Input: dimensioned drawing with shaded views. Units: mm. Origin: part minimum x, y, z. Coordinates: 2 decimals unless noted, no trailing zeros. Order: outer loops, then holes, each group sorted by start corner. A loop starts at its lowest first (then second) coordinate and runs counter-clockwise, first axis right, second up.
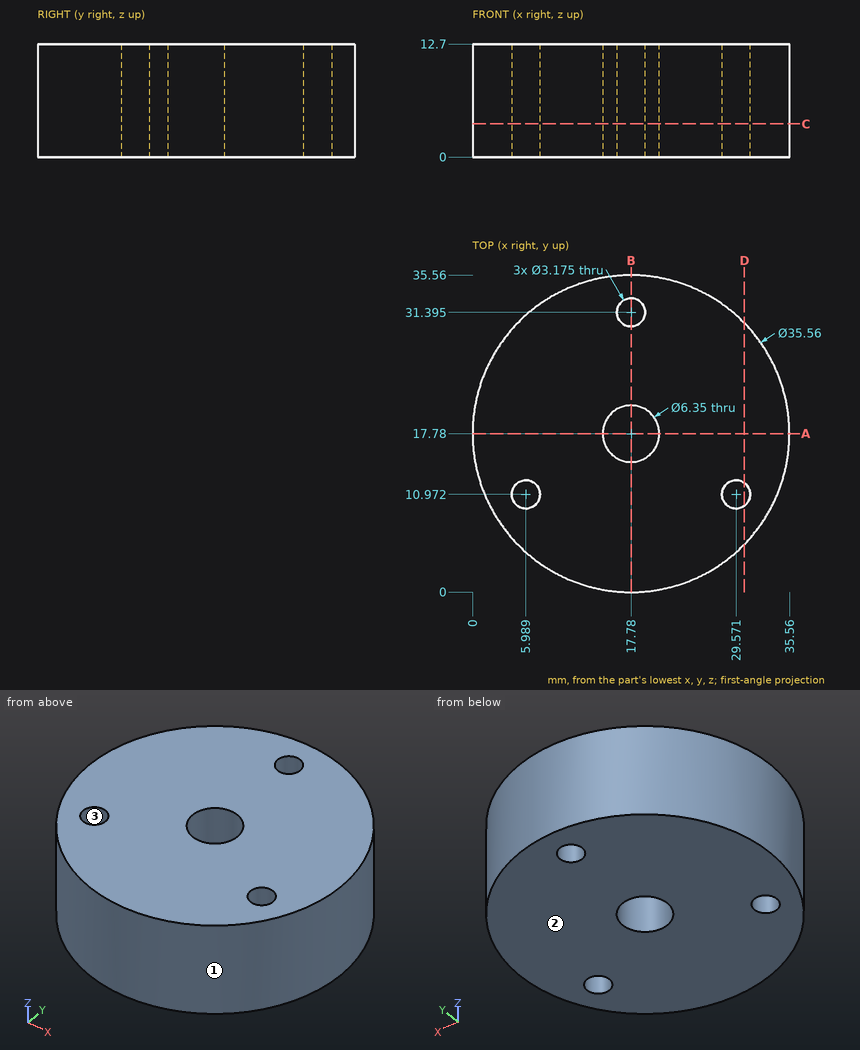
1. Section query A-A on y = 17.78. Return loops of the section in (x, z) (1 decimal), plus the area to 3 significant figures.
Findings:
outline: (0, 0) - (14.6, 0) - (14.6, 12.7) - (0, 12.7) - close; (21, 0) - (35.6, 0) - (35.6, 12.7) - (21, 12.7) - close
area: 371 mm2
2. Section query C-C on z = 3.75. Count the separate pieces of the cut face and the enclosed holes in it, plus the area to 3 significant figures.
Findings:
separate pieces: 1
enclosed holes: 4
area: 938 mm2
3. Pin query (flat end, axial travel): P1, Ø4, axis at x = 4.5, z = 3.5, coming from the +Y side; P2, Ø3, axis at x = 29.57, y = 10.97, coming from the -Z side. Return the tip coordinate at first contact, or that it passes through.
Findings:
P1: stops at y = 31.52
P2: passes through
4. Draft query along X for the marked faces 1, 2 and 3. Return one class per face: released by +X, released by -X, zero draft, split by the parting line, or undercut.
Findings:
face 1: split by the parting line
face 2: zero draft
face 3: undercut
5. Section query D-D on x = 30.5. Return loops of the section in (y, z) (1 decimal).
Findings:
outline: (5.4, 0) - (9.7, 0) - (9.7, 12.7) - (5.4, 12.7) - close; (12.3, 0) - (30.2, 0) - (30.2, 12.7) - (12.3, 12.7) - close
6. Section query B-B on x = 17.78. Return loops of the section in (y, z) (1 decimal).
Findings:
outline: (0, 0) - (14.6, 0) - (14.6, 12.7) - (0, 12.7) - close; (21, 0) - (29.8, 0) - (29.8, 12.7) - (21, 12.7) - close; (33, 0) - (35.6, 0) - (35.6, 12.7) - (33, 12.7) - close
7. Ray query, line 1 (Y direction, x = 17.78, z = 4.25) (1 decimal); line 2 (X direction, y = 18, z = 3); line 3 (X direction, y = 12, z = 3.25) (1 decimal). Return the intervals inside material, ascending.
Findings:
line 1: y = 0 to 14.6, 21 to 29.8, 33 to 35.6
line 2: x = 0 to 14.61, 20.95 to 35.56
line 3: x = 1 to 4.8, 7.2 to 28.4, 30.8 to 34.6
